Read the model definition and answer for the solid it produces. Units are mm, in the model's axes. Face numbers are marked on the shaded views. A direction names the side the tool comes from. Round coordinates to 2 decimals unless told otherwise and drop trailing zeros. Loops run counter-clockwise (first coordinate to the right, second up) from the corner with the lowest first, then second, coordinate; pieces in that order, holes last. Notation, with made-up numbers: (64, -14.5) -> (79, -14.5) arc R18 ccw to (79, -8.5) -> close; hole circle Ø9 at (81.5, 46.5). An arc over 180 degrees is marked (long way). Put each result on its own line as item: value.
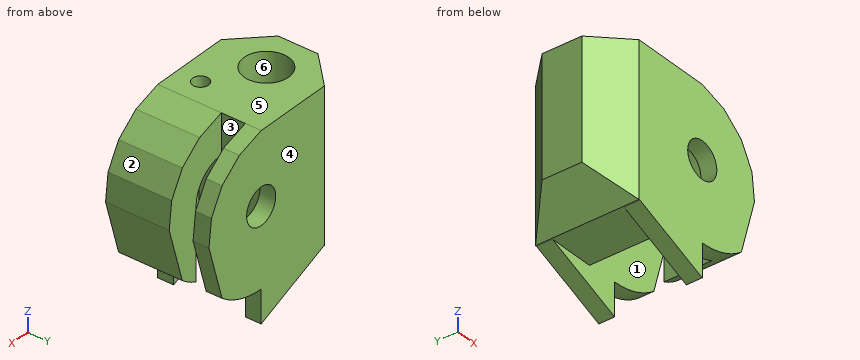
Autodesk Inventor part; units mm, degrees
ref_plane "YZ Plane" through (0, 0, 0) normal (1, 0, 0) x (0, 1, 0)
ref_plane "XZ Plane" through (0, 0, 0) normal (0, 1, 0) x (-1, 0, 0)
ref_plane "XY Plane" through (0, 0, 0) normal (0, 0, 1) x (1, 0, 0)
sketch "スケッチ1" plane through (0, 0, 0) normal (0, 1, 0) x (-1, 0, 0)
  circle A0 centre (0, 0) radius 1.15
  circle A1 centre (0, 0) radius 2
  circle A2 centre (0, 0) radius 5
  line L0 (0, 0) -> (7, 0)
  line L1 (7, 0) -> (7, 4.5)
  line L2 (7, 4.5) -> (0, 4.5)
  line L3 (0, 4.5) -> (0, 0)
  line L4 (0, 0) -> (7, 0)
  line L5 (7, 0) -> (7, -5)
  line L6 (7, -5) -> (0, -5)
  line L7 (0, -5) -> (0, 0)
  line L8 (0, 4.5) -> (-2, 4.5)
  line L9 (-2, 4.5) -> (-2, 0)
  line L10 (-2, 0) -> (0, 0)
  line L11 (0, 0) -> (0, 4.5)
  circle A3 centre (0, 0) radius 3
  line L12 (-2, 0) -> (-2, -5)
  line L13 (-2, -5) -> (0, -5)
  line L14 (2, 0) -> (2, -5)
  circle A4 centre (0, 0) radius 4.9244
  line L15 (-2, 0) -> (-4.9244, 0)
  line L16 (0, -4.9244) -> (0, -5.9244)
  line L17 (0, -5.9244) -> (7, -5.9244)
  line L18 (7, -5.9244) -> (7, -5)
  line L19 (7, -5) -> (0, -5.9244)
  line L20 (0, -5.9244) -> (4.9138, -5)
  line L21 (0, -5) -> (0, -7)
  line L22 (0, -7) -> (4.9138, -5)
  point P0 (0, 2)
  point P1 (-2, 2.2361)
  point P2 (-2, -2.2361)
  point P3 (-2, -4.5826)
  point P4 (-2, -4.5)
  point P5 (0, -4.9244)
  dimension "d2" = 10
  dimension "d0" = 2.3
  dimension "d1" = 4
  dimension "d3" = 7
  dimension "d4" = 4.5
  dimension "d5" = 6
  dimension "d22" = 1
  dimension "d34" = 5
  dimension "d39" = 2
extrude "押し出し1" add sketch "スケッチ1" along normal blind 4.5 contours A1 L3 A3 L0 | L0 A3 L14 | A3 L3 L2 A4 L0 | L0 A4 L14 A3 | A4 L2 A2 L0 | L0 A2 L14 A4 | L0 L5 L6 L14 A2 | A2 L2 L1 L0
extrude "押し出し2" add sketch "スケッチ1" along normal blind 3 contours A1 L9 A3 L3 | L15 A3 L9 | L12 A3 L15 | A3 L9 L8 L3 | A3 L15 A4 L9 | L12 A4 L15 A3
extrude "押し出し3" add sketch "スケッチ1" against normal blind 1 contours L0 A1 L7 A0 | A0 L3 A1 L0 | A0 L10 A1 L3 | L7 A1 L10 A0 | L14 A3 L7 A1 | A1 L3 A3 L0 | L0 A3 L14 | A1 L9 A3 L3 | L7 A3 L12 A1 | A3 L3 L2 A4 L0 | L0 A4 L14 A3 | L14 A4 L7 A3 | L15 A3 L9 | L12 A3 L15 | A3 L9 L8 L3 | L7 A4 L12 A3 | A4 L2 A2 L0 | L0 A2 L14 A4 | L14 A2 L7 A4 | A3 L15 A4 L9 | L12 A4 L15 A3 | L0 L5 L6 L14 A2 | A2 L2 L1 L0 | L14 L6 A2 | L6 L20 L16 | L19 L22 L17 | L20 L22 L19 | L17 L22 L21
sketch "スケッチ2" plane through (0, 4.5, 0) normal (0, 1, 0) x (1, 0, 0)
  circle A0 centre (0, 0) radius 1.15
  circle A1 centre (0, 0) radius 2
  circle A2 centre (0, 0) radius 4.9244
  line L0 (0, 0) -> (2, 0)
  line L1 (2, 0) -> (2, -4.5)
  line L2 (2, -4.5) -> (0, -4.5)
  line L3 (0, -4.5) -> (0, 0)
  line L4 (-2, 5) -> (-7, 5)
  line L5 (0, -4.5) -> (-7, -4.5)
  line L6 (-7, -4.5) -> (-7, 5)
  line L7 (-7, 5) -> (0, 5)
  line L8 (0, 5) -> (0, -4.5)
  line L9 (0, 0) -> (2, 0)
  line L10 (2, 0) -> (2, 5)
  line L11 (2, 5) -> (0, 5)
  line L12 (0, 5) -> (0, 0)
  line L13 (0, 5) -> (-7, 5)
  line L14 (0, 5.9244) -> (0, 5)
  line L15 (-7, 5) -> (0, 5.9244)
  line L16 (0, 5.9244) -> (-4.9138, 5)
  line L17 (-2, 5) -> (-7, 5)
  line L18 (0, 5) -> (0, 7)
  line L19 (0, 7) -> (-4.9138, 5)
  point P0 (0, 4.9244)
  dimension "d12" = 4
  dimension "d35" = 5
  dimension "d40" = 2
extrude "押し出し4" add sketch "スケッチ2" along normal blind 1 contours L0 A1 L3 A0 | A0 L8 A1 L0 | A0 L3 A1 L8 | L1 L2 L3 A1 | L10 A2 L1 | A1 L8 A2 L10 | A1 L3 L5 A2 L8 | A2 L5 L6 L4 L7 L8 | L7 L4 L16 L14 | L16 L19 L15 | L15 L19 L18
sketch "スケッチ4" plane through (0, 3, 4.5) normal (0, 0, 1) x (1, 0, 0)
  line L0 (-7, 2.5) -> (2, 2.5)
  line L1 (-7, 2.5) -> (-4.5, 2.5)
  line L2 (-4.5, 2.5) -> (-4.5, -0.75)
  line L3 (-4.5, -0.75) -> (-7, -0.75)
  line L4 (-7, -0.75) -> (-7, 2.5)
  circle A0 centre (-4.5, -0.75) radius 1.4
  line L5 (0, -3) -> (0, -2.5)
  line L6 (0, -2.5) -> (-1.5, -2.5)
  circle A1 centre (-1.5, -2.5) radius 0.5
  dimension "d23" = 2.5
  dimension "d24" = 3.25
  dimension "d25" = 2.8
  dimension "d26" = 0.5
  dimension "d27" = 1.5
  dimension "d28" = 1
extrude "押し出し6" cut sketch "スケッチ4" against normal blind 6 contours A0 L3 L2 | L2 L3 A0 | A1
chamfer "面取り2" distance 2 angle 45 3 edges at (-7, 5.5, -0.25) (-7, -1, -0.25) (-7, 2.25, -5)
chamfer "面取り3" distance 2 angle 45 2 edges at (2, 5, 4.5) (2, 1, 4.5)
chamfer "面取り4" distance 2 angle 45 2 edges at (3.6246, 5, 3.3335) (3.6246, 1, 3.3335)
chamfer "面取り5" distance 2 angle 45 2 edges at (4.6513, 1, 1.6172) (4.6513, 5, 1.6172)
chamfer "面取り6" distance 2 angle 45 2 edges at (4.9108, 1, -0.3659) (4.9108, 5, -0.3659)
chamfer "面取り7" distance 2 angle 45 2 edges at (4.3603, 5, -2.2887) (4.3603, 1, -2.2887)
properties part number "rod5.7"
Item 1: The part is cut by section B-B (y = 4.25). Determine the outline of the cut face in (x, z).
Derived:
outline: (-6.25, -3.75) -> (-5, -5) -> (-2, -5) -> (-2, 0) arc R2 cw to (0, 2) -> (0, 4.5) -> (-6.25, 4.5) -> close
Item 2: Which of the six approach directions +Z, -Z, +X, -X, +Y, -Y give full straight-line access (tool end or side, diameter ignored) to the marked faces 1, 2 and 3?
Derived:
face 1: -Z, +X
face 2: +Z, +X, +Y, -Y
face 3: +Z, -Z, +X
Item 3: Flat-ended cylindrical pins translate along their axes: pin 1 Ø3 at (y, z) = (0, -2) entering from +X; pin 2 Ø0.8 at (y, z) = (5, -5.5) entering from +X; pin 3 Ø2 at (x, y) = (2.5, 4.5) entering from +Z. Find the tip coordinate at first contact, or state that the pin passes through.
Derived:
pin 1: stops at x = 4.07
pin 2: stops at x = 0
pin 3: stops at z = 4.02
Item 4: For a pull along Y with two mould halves and no side action, classify the marked faces 4, 5 and 6 as pulls with the +Y half, pulls with the -Y half, needs draft (parallel to the pull), parting line crosses it, or undercut.
Derived:
face 4: pulls with the +Y half
face 5: needs draft
face 6: undercut
Item 5: The part is cut by section D-D (x = 0.75). Determine the outline of the cut face in (y, z), then the cut area to 3 significant figures.
Derived:
outline: (-1, -4.87) -> (0, -4.87) -> (0, -0.87) -> (-1, -0.87) -> close; (-1, 0.87) -> (0, 0.87) -> (0, 1.85) -> (3, 1.85) -> (3, 4.26) -> (-1, 4.26) -> close; (4.5, -4.87) -> (5.5, -4.87) -> (5.5, -0.87) -> (4.5, -0.87) -> close; (4.5, 0.87) -> (5.5, 0.87) -> (5.5, 4.26) -> (4.5, 4.26) -> close
area: 22.0 mm^2
Item 6: The part is cut by section C-C (z = -6). Determine the outline of the cut face in (x, y).
Derived:
outline: (-2.46, -1) -> (0, -1) -> (0, 0) -> (-2.46, 0) -> close; (-2.46, 4.5) -> (0, 4.5) -> (0, 5.5) -> (-2.46, 5.5) -> close
Item 7: Find the intervals of material crossed by line 1 along Y through (x, z) = (-4.5, 1.1); line 2 along X through (y, z) = (2.25, 0.25); line 3 along Y through (x, z) = (-1.5, 3.15), in increasing order.
Derived:
line 1: y = -1 to 0.85, 3.65 to 5.5
line 2: x = -7 to -5.9, -3.1 to -1.98, 1.98 to 4.06
line 3: y = -1 to 0, 1 to 5.5
Item 8: The part is cut by section A-A (x = -0.5). Determine the outline of the cut face in (y, z), then the cut area to 3 significant figures.
Derived:
outline: (-1, -6.8) -> (0, -6.8) -> (0, -1.04) -> (-1, -1.04) -> close; (-1, 1.04) -> (0, 1.04) -> (0, 1.94) -> (4.5, 1.94) -> (4.5, 1.04) -> (5.5, 1.04) -> (5.5, 4.5) -> (-1, 4.5) -> close; (4.5, -6.8) -> (5.5, -6.8) -> (5.5, -1.04) -> (4.5, -1.04) -> close
area: 30.0 mm^2
